from build123d import *

# Parameters (mm, degrees)
F1_DEPTH    = 70
F2_T1_DEPTH = 70
F3_T1_DEPTH = 70
F5_DEPTH    = 15
F6_SIZE     = 9
F7_R        = 9
F8_DEPTH    = 3
F9_R        = 5
F10_DEPTH   = 25
F11_R       = 10
F11_R_2     = 5
F12_DEPTH   = 2


# Not quite as in the source:
# - a fillet or chamfer that OpenCascade refuses, or shapes differently, is made with other operations: its cross-section is extruded or revolved along the edge and cut away or added


with BuildPart() as f1:
    # F0 (on Front) → F1 (new body)
    with BuildSketch(Plane.XZ):
        with BuildLine():
            Line((45, -5), (17.2916164658, -5))
            ThreePointArc((17.2916164658, -5), (10.8166538264, -14.3874945699), (0, -18))
            Line((0, -18), (0, -20))
            Line((0, -20), (45, -20))
            Line((45, -20), (45, -5))
        make_face()
        with BuildLine():
            ThreePointArc((17.2916164658, -5), (17.8220242451, -2.5249657043), (18, 0))
            ThreePointArc((18, 0), (-2.5249657043, 17.8220242451), (-17.2916164658, -5))
            ThreePointArc((-17.2916164658, -5), (-10.8166538264, -14.3874945699), (0, -18))
            ThreePointArc((0, -18), (10.8166538264, -14.3874945699), (17.2916164658, -5))
        make_face()
        with BuildLine():
            ThreePointArc((9, 0), (6.3639610307, -6.3639610307), (0, -9))
            ThreePointArc((0, -9), (-6.3639610307, 6.3639610307), (9, 0))
        make_face(mode=Mode.SUBTRACT)
        with BuildLine():
            ThreePointArc((0, -18), (-10.8166538264, -14.3874945699), (-17.2916164658, -5))
            Line((-17.2916164658, -5), (-45, -5))
            Line((-45, -5), (-45, -20))
            Line((-45, -20), (0, -20))
            Line((0, -20), (0, -18))
        make_face()
    extrude(amount=F1_DEPTH)

    # F2: fillet of radius 5 on 1 edges, made by hand

    # F2_s2 → F2_t1 (join)
    with BuildSketch(Plane.XZ):
        with BuildLine():
            ThreePointArc((-18, 0), (-19.4644660941, -3.5355339059), (-23, -5))
            Line((-23, -5), (-17.2916164658, -5))
            ThreePointArc((-17.2916164658, -5), (-17.8220242451, -2.5249657043), (-18, 0))
        make_face()
    extrude(amount=F2_T1_DEPTH)

    # F3: fillet of radius 5 on 1 edges, made by hand

    # F3_s2 → F3_t1 (join)
    with BuildSketch(Plane.XZ):
        with BuildLine():
            ThreePointArc((23, -5), (19.4644660941, -3.5355339059), (18, 0))
            ThreePointArc((18, 0), (17.8220242451, -2.5249657043), (17.2916164658, -5))
            Line((17.2916164658, -5), (23, -5))
        make_face()
    extrude(amount=F3_T1_DEPTH)

    # F4 (on Front) → F5 (join)
    with BuildSketch(Plane.XZ):
        with BuildLine():
            Line((23, -5), (45, -5))
            Line((45, -5), (45, 50))
            Line((45, 50), (-45, 50))
            Line((-45, 50), (-45, -5))
            Line((-45, -5), (-23, -5))
            ThreePointArc((-23, -5), (-19.4644660941, -3.5355339059), (-18, 0))
            ThreePointArc((-18, 0), (0, 18), (18, 0))
            ThreePointArc((18, 0), (19.4644660941, -3.5355339059), (23, -5))
        make_face()
    extrude(amount=F5_DEPTH)

    # F6
    f6_edges = [f1.edges().sort_by_distance(p)[0] for p in [
        (45, -7.5, 50),
        (-45, -7.5, 50),
    ]]
    chamfer(f6_edges, length=F6_SIZE)

    # F7 (on face) → F8 (join)
    with BuildSketch(Plane.XZ.offset(70)):
        with BuildLine():
            ThreePointArc((-18, 0), (0, -18), (18, 0))
            ThreePointArc((18, 0), (0, 18), (-18, 0))
        make_face()
        Circle(F7_R, mode=Mode.SUBTRACT)
    extrude(amount=F8_DEPTH)

    # F9 (on face) → F10 (cut)
    with BuildSketch(Plane.XZ.offset(15)):
        with Locations((0, 38)):
            Circle(F9_R)
    extrude(amount=-F10_DEPTH, mode=Mode.SUBTRACT)

    # F11 (on face) → F12 (join)
    with BuildSketch(Plane.XZ.offset(15)):
        with Locations((0, 38)):
            Circle(F11_R)
        with Locations((0, 38)):
            Circle(F11_R_2, mode=Mode.SUBTRACT)
    extrude(amount=F12_DEPTH)


solid = f1.part
Read the model definition and answer for the solid it produces. Units are mm, in the model's axes. A direction names the side the tool comes from. Coordinates: 2 decimals unless noted, no trailing zeros. Loops run counter-clockwise (first coordinate to the right, second up) from the corner with the lowest first, then second, coordinate; pieces in that order, holes last.
Q1. Which of the six approach directions +Z, -Z, +X, -X, +Y, -Y give full straight-line access (tool end or side, diameter ignored) to faces 1 (the face through (-5, -17, 36)), 2 (the face through (-19, -42, -3)), 3 (the face through (34, -42, -5))?
Q2. The part is cut by section A-A on z = 38. Write down the section's boundary in (x, y).
Q3. Each of these flat-tipped pins is pushed along its axis until it touches: pin 1 Ø1.5 at (y, z) = (-63.5, 20.5) entering from +X; pin 2 Ø24 at (x, y) = (-39, -41) entering from +Z; pin 3 Ø5 at (y, z) = (-21, 12.5) entering from +X; pin 4 Ø22 at (x, z) = (4, 43) entering from -Y. Where does it stop, or does it pass through?
Q4. The mould has two halves that part along Z. Classify faces 4 (the face through (20, -42, -4)), 5 (the face through (-45, -19, -9)), 6 (the face through (-2.17, -15.99, 28.24)): +Z half, -Z half, draft (parallel to the pull), parting line (faces both ways), or undercut.
Q5. The part is cut by section B-B on y = -11. Write down the section's boundary in (x, z).
Q6. The part is cut by section D-D on x = -34.5. Write down the section's boundary in (y, z), and give its area (4 significant figures).
Q7. The part is cut by section C-C on y = -48.5. Write down the section's boundary in (x, z).
Q8. Consider probe 1 along Z at (x, y) = (-39, -68); probe 2 along Y at (x, z) = (8, 29); probe 3 along X at (y, z) = (-10, 6). Determine where each line is inside the solid, lowest interval first.
Results below:
1. face 1: +Z, +X, -X, -Y
1. face 2: +Z, -X, -Y
1. face 3: +Z, +X, -Y
2. outline: (-45, -15) - (-10, -15) - (-10, -17) - (-5, -17) - (-5, 0) - (-45, 0) - close; (5, -17) - (10, -17) - (10, -15) - (45, -15) - (45, 0) - (5, 0) - close
3. pin 1: passes through
3. pin 2: stops at z = -5
3. pin 3: stops at x = 14.97
3. pin 4: stops at y = -17
4. face 4: +Z half
4. face 5: draft
4. face 6: undercut
5. outline: (-45, -20) - (45, -20) - (45, 41) - (36, 50) - (-36, 50) - (-45, 41) - close; hole circle Ø18 at (0, 0); hole circle Ø10 at (0, 38)
6. outline: (-70, -20) - (0, -20) - (0, 50) - (-15, 50) - (-15, -5) - (-70, -5) - close
6. area: 1,875 mm2
7. outline: (-45, -20) - (45, -20) - (45, -5) - (23, -5) arc R5 cw to (18, 0) arc R18 ccw to (-18, 0) arc R5 cw to (-23, -5) - (-45, -5) - close; hole circle Ø18 at (0, 0)
8. probe 1: z = -20 to -5
8. probe 2: y = -15 to 0
8. probe 3: x = -45 to -6.71, 6.71 to 45
